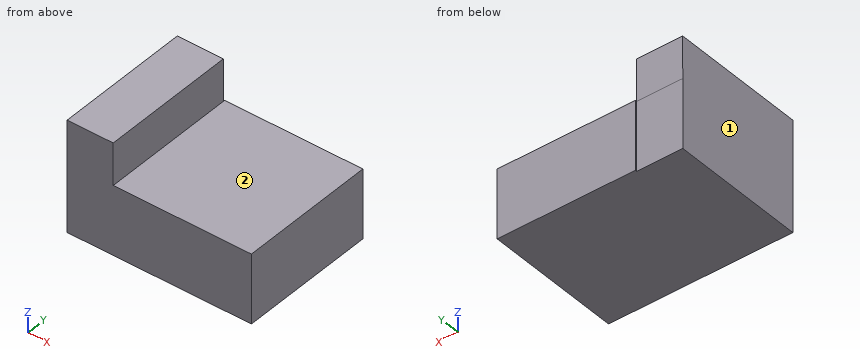
```python
from build123d import *

# Parameters (mm, degrees)
F0_W     = 38.1
F0_H     = 38.1
F1_DEPTH = 19.05
F3_DEPTH = 12.7
F4_DEPTH = 19.05


with BuildPart() as f1:
    # F0 (on Top) → F1 (new body)
    with BuildSketch(Plane.XY):
        with Locations((-2.1893925067, -1.1373543657)):
            Rectangle(F0_W, F0_H)
    extrude(amount=F1_DEPTH)



with BuildPart() as f3:
    # F2 (on face) → F3 (new body)
    with BuildSketch(Plane(origin=(-21.2393925067, 0, 0), x_dir=(0, -1, 0), z_dir=(-1, 0, 0))):
        Polygon((-17.4572191403, 19.05), (20.1873543657, 19.05), (20.1873543657, 30.6271831505), (-17.4629575457, 30.6271831505), align=None)
    extrude(amount=F3_DEPTH)


with BuildPart() as f1_1:
    add(f1.part)
    # F4 (add): a face of the model
    f4_faces = [f3.part.faces().sort_by_distance(p)[0] for p in [
        (-27.5893925067, -1.3650676127, 19.05),
    ]]

    add(f3.part)  # F4 merges F3
    extrude(f4_faces, amount=F4_DEPTH)


solid = f1_1.part
```
Source: CAD feature listing. Evaluate the final solid. Frame: model axes, mm. Face numbers are marked on the shaded views. A direction names the side the tool comes from. Coordinates: 2 decimals unless noted, no trailing zeros. Write each loop counter-clockwise with the first axis right and the second up, starting at its lowest first coordinate (ties: lowest second). Pieces come first, ordered by that corner, then holes. Notation, with made-up numbers: (26.25, -14) - (58.25, -14) arc R9 cw to (58.25, 0) - close; hole circle Ø3 at (57, 42). An arc over 180 degrees is marked (long way). Answer as a JSON object with one key per item and string values.
Q1. Section query C-C, the plane z = 26. Output: boundary loops of the cut face in (x, y), plus the area to 3 significant figures.
Ans:
{"outline": "(-33.94, -20.19) - (-21.24, -20.19) - (-21.24, 17.46) - (-33.94, 17.46) - close", "area": "478 mm2"}
Q2. First-contact query: pin 1 Ø19 at (x, y) = (6, 1) entering from +Z; pin 2 Ø10 at (x, z) = (-27, 13) entering from +Y. Flat tips, straight axial feed; report the tip coordinate or a pass-through.
Ans:
{"pin 1": "stops at z = 19.05", "pin 2": "stops at y = 17.46"}
Q3. Set-up query: the marked faces 1 and 2. Return all of +Z, -Z, +X, -X, +Y, -Y with unobstructed straight access to the full face (end or side cutting, diameter ignored); none if empty.
Ans:
{"face 1": "+Z, -Z, -X, +Y, -Y", "face 2": "+Z, +X, +Y, -Y"}
Q4. Material intervals for line 1 (X direction, y = -11.5, z = 22); line 2 (Y direction, x = -32, z = 10); line 3 (Z direction, x = 2, y = 5.5), sorted ascending. Write a range as [from, to].
Ans:
{"line 1": "x = [-33.94, -21.24]", "line 2": "y = [-20.19, 17.46]", "line 3": "z = [0, 19.05]"}
Q5. Section query B-B, the plane x = -0.5. Output: boundary loops of the cut face in (y, z), plus the area to 3 significant figures.
Ans:
{"outline": "(-20.19, 0) - (17.91, 0) - (17.91, 19.05) - (-20.19, 19.05) - close", "area": "726 mm2"}
Q6. Section query A-A, the plane y = 4.5. Output: boundary loops of the cut face in (x, z), plus the area to 3 significant figures.
Ans:
{"outline": "(-33.94, 0) - (16.86, 0) - (16.86, 19.05) - (-21.24, 19.05) - (-21.24, 30.63) - (-33.94, 30.63) - close", "area": "1,110 mm2"}
